Answer from the drawing. Dimensions are ordinates in mm from the lowest x, y and z of the part. Round coordinates to 2 decimals unless told otherwise and drop trailing zeros. Write each loop counter-clockwise with the first axis right and the second up, starting at its lowest first coordinate (ties: lowest second). Pieces come first, ordered by that corner, then holes.
1. Flat-ended cylindrical pins translate along their axes: pin 1 Ø10 at (y, z) = (11.5, 10.5) entering from +X; pin 2 Ø3 at (y, z) = (16.5, 3) entering from -X; pin 3 Ø4.5 at (x, y) = (2.5, 75.23) entering from -Z; pin 4 Ø5 at (x, z) = (31, 9.5) entering from -Y. Find the tip coordinate at first contact, or state that the pin passes through.
2. Straight lines are drawn through the part: probe 1 along Y at (x, z) = (2.5, 15.1); probe 2 along X at (y, z) = (2.5, 15.7); probe 3 along Z at (x, y) = (11, 25). For each, find the intervals that lie inside material, in ascending order.
3. Find section A-A (y = 2.5). Write down the section's boundary in (x, z).
4. Find section B-B (x = 22). Write down the section's boundary in (y, z), and give its area (3 significant figures).
5. Determine the mould class of the marked faces 1 and 2 for opening direction X: pulls with the +X half, pulls with the -X half, needs draft (parallel to the pull), parting line crosses it, or undercut.
6. Find section C-C (z = 2.5). Count the separate pieces of the cut face and the enclosed holes in it.
7. Find section D-D (y = 56.5). Write down the section's boundary in (x, z).
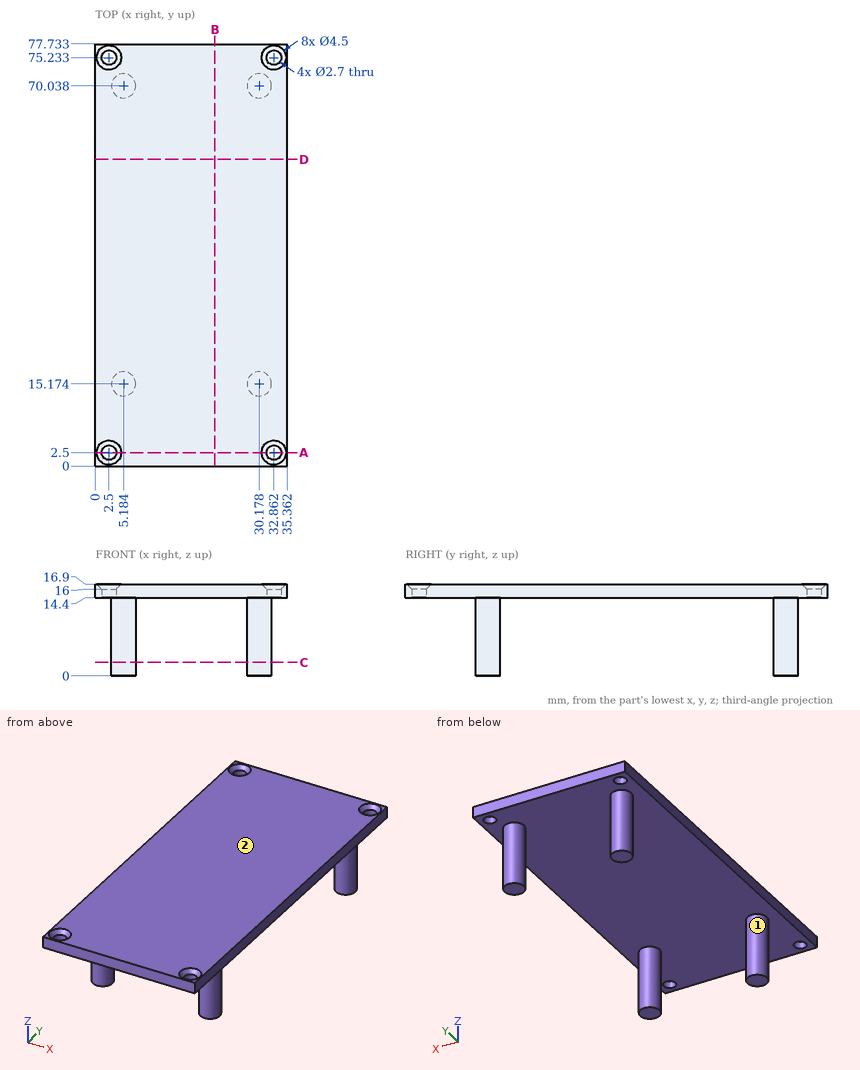
Worked answers:
1. pin 1: stops at x = 35.36
1. pin 2: stops at x = 2.93
1. pin 3: stops at z = 14.4
1. pin 4: stops at y = 12.92
2. probe 1: y = 0 to 1.15, 3.85 to 73.88, 76.58 to 77.73
2. probe 2: x = 0 to 1.15, 3.85 to 31.51, 34.21 to 35.36
2. probe 3: z = 14.4 to 16.9
3. outline: (0, 14.4) - (1.15, 14.4) - (1.15, 16) - (0.25, 16.9) - (0, 16.9) - close; (3.85, 14.4) - (31.51, 14.4) - (31.51, 16) - (30.61, 16.9) - (4.75, 16.9) - (3.85, 16) - close; (34.21, 14.4) - (35.36, 14.4) - (35.36, 16.9) - (35.11, 16.9) - (34.21, 16) - close
4. outline: (0, 14.4) - (77.73, 14.4) - (77.73, 16.9) - (0, 16.9) - close
4. area: 194 mm2
5. face 1: undercut
5. face 2: needs draft
6. separate pieces: 4
6. enclosed holes: 0
7. outline: (0, 14.4) - (35.36, 14.4) - (35.36, 16.9) - (0, 16.9) - close
